from build123d import *

# Parameters (mm, degrees)
F0_W     = 14.142123667
F0_H     = 50.8
F1_DEPTH = 14.732
F2_R     = 2.54
F3_R     = 0.79375
F4_R     = 4.4176924247
F4_W     = 4.9146201927
F4_H     = 3.3284204943
F5_DEPTH = 38.1


with BuildPart() as f1:
    # F0 (on Top) → F1 (new body)
    with BuildSketch(Plane.XY):
        Polygon((10.7273911178, 53.3604013813), (-7.1363440174, 22.8804013813), (7.0057796496, 22.8804013813), align=None)
        with Locations((-0.0652821839, -2.5195986187)):
            Rectangle(F0_W, F0_H)
        Polygon((7.0057796496, -27.9195986187), (-7.1363440174, -27.9195986187), (-13.0909229835, -46.1554975013), (17.6123739426, -46.1554975013), align=None)
    extrude(amount=F1_DEPTH)

    # F2
    f2_edges = [f1.edges().sort_by_distance(p)[0] for p in [
        (7.00578, -27.919599, 7.366),
        (7.00578, 22.880401, 7.366),
        (-13.090923, -46.155498, 7.366),
        (17.612374, -46.155498, 7.366),
        (-7.136344, 22.880401, 7.366),
        (-7.136344, -27.919599, 7.366),
    ]]
    fillet(f2_edges, radius=F2_R)

    # F3
    f3_edges = [f1.edges().sort_by_distance(p)[0] for p in [
        (10.727391, 53.360401, 7.366),
    ]]
    fillet(f3_edges, radius=F3_R)

    # F4 (on face) → F5 (cut)
    with BuildSketch(Plane.XY.offset(14.732)):
        with Locations((0, -24.7696824372)):
            Circle(F4_R)
        Polygon((-1.2388014392, 28.897959739), (-4.5963440174, 22.1909237022), (-4.5963440174, -19.0687216818), (-1.2388014392, -15.5301969498), align=None)
        Polygon((1.3100893161, 33.960372903), (1.3100893161, 28.550172903), (1.3100893161, -16.671693043), (4.8148863068, -20.562165355), (4.8148863068, 22.7259079205), (7.4699121839, 44.4705713353), align=None)
        Polygon((-8.5027228454, -42.827077007), (-9.5895539796, -46.1554975013), (-5.5043729953, -46.1554975013), (-5.5043729953, -42.827077007), align=None)
        with Locations((0.2948777983, -44.4912872541)):
            Rectangle(F4_W, F4_H)
        Polygon((6.2907133251, -42.827077007), (6.2907133251, -46.1554975013), (13.1966339, -46.1554975013), (10.6155779213, -42.827077007), align=None)
    extrude(amount=-F5_DEPTH, mode=Mode.SUBTRACT)


solid = f1.part
Verification items for the finished model (mm, model axes). A direction names the side the tool comes from. Give positions to 0.01 mm unless a question says otherwise; leave off trailing zeros. Loops run counter-clockwise (first coordinate to the right, second up) from the corner with the lowest first, then second, coordinate; pieces in that order, holes last.
1) Sectioned sample at D-D, the plane y = 37. Enter the section's corners in (x, z).
2) Sectioned sample at C-C, the plane x = 0. Enter the section's corners in (y, z).
3) Sectioned sample at A-A, the plane y = -12.5. Enter the section's corners in (x, z), then the cut area to 3 significant figures.
4) Thickness scan on line 1 along X through (y, z) = (-6, 1.25); line 2 along Y through (x, z) = (-1.5, 9); line 3 along Y through (x, z) = (-3.5, 13.5). Record the ranges inside material, lowest first.
5) Depth check by flat-ended pin: pin 1 Ø2.5 at (y, z) = (-45, 9.5) entering from +X; pin 2 Ø2 at (x, z) = (6.5, 7) entering from +Y; pin 3 Ø8 at (x, y) = (0, -24.77) entering from +Z; pin 4 Ø8 at (x, y) = (0.5, 32) entering from -Z. Enter the tip coordinate at first touch or a pass-through.
6) Set-up check for faces 5 (the flat face through (4.815, 1, 7)), 6 (the flat face through (7.006, -3, 7)), 7 (the flat face through (-7.136, -3, 7)), 8 (the flat face through (-4, -46.155, 7)), 9 (the flat face through (-7, -42.827, 7)): record each of +Z, -Z, +X, -X, +Y, -Y from which the full face is reachable in a straight line by a thin tool's end or side.
7) Draft check along X on faces 1 (the flat face through (-9.6, -35.46, 7.26)), 2 (the flat face through (4, -46.155, 7)), 3 (the flat face through (3.04, -18.59, 7.47)), 4 (the flat face through (-2.941, -17.324, 7.469)). Enter one of: pulls with the +X half, pulls with the -X half, needs draft (parallel to the pull), parting line crosses it, or undercut.
8) Sectioned sample at B-B, the plane z = 8.25. Count the separate pieces of the cut face and the enclosed holes in it, then the cut area to 3 significant figures.
Answers:
1. outline: (1.14, 0) - (3.09, 0) - (3.09, 14.73) - (1.14, 14.73) - close; (6.56, 0) - (8.73, 0) - (8.73, 14.73) - (6.56, 14.73) - close
2. outline: (-42.83, 0) - (-29.19, 0) - (-29.19, 14.73) - (-42.83, 14.73) - close; (-20.35, 0) - (35.06, 0) - (35.06, 14.73) - (-20.35, 14.73) - close
3. outline: (-7.14, 0) - (-4.6, 0) - (-4.6, 14.73) - (-7.14, 14.73) - close; (-1.24, 0) - (1.31, 0) - (1.31, 14.73) - (-1.24, 14.73) - close; (4.81, 0) - (7.01, 0) - (7.01, 14.73) - (4.81, 14.73) - close
3. area: 107 mm2
4. line 1: x = -7.14 to -4.6, -1.24 to 1.31, 4.81 to 7.01
4. line 2: y = -42.83 to -28.92, -20.61 to -15.81, 28.38 to 32.5
4. line 3: y = -46.16 to -27.47, -22.07 to -17.91, 24.38 to 29.08
5. pin 1: stops at x = 15.73
5. pin 2: stops at y = 47.85
5. pin 3: passes through
5. pin 4: stops at z = 0
6. face 5: +Z, -Z
6. face 6: +Z, -Z, +X
6. face 7: +Z, -Z, -X, +Y
6. face 8: +Z, -Z, +X, -X, -Y
6. face 9: +Z, -Z, -Y
7. face 1: pulls with the -X half
7. face 2: needs draft
7. face 3: undercut
7. face 4: undercut
8. separate pieces: 1
8. enclosed holes: 3
8. area: 864 mm2
